```python
from build123d import *

# Parameters (mm, degrees)
SKETCH1_W           = 50
SKETCH1_H           = 50
BOSS_EXTRUDE1_DEPTH = 10
CUT_EXTRUDE3_DEPTH  = 6.3
SKETCH5_R           = 6.5
SKETCH5_R_2         = 3.1
BOSS_EXTRUDE2_DEPTH = 0.5
CUT_EXTRUDE4_DEPTH  = 57.789083458
FILLET2_R           = 5
CHAMFER2_SIZE       = 1
CHAMFER2_SIZE2      = 1.414213562
FILLET3_R           = 2
SKETCH9_R           = 3.1
CUT_EXTRUDE5_DEPTH  = 36.912254176
CHAMFER3_SIZE       = 1
SKETCH10_W          = 52
SKETCH10_H          = 19.709433282
CUT_EXTRUDE6_DEPTH  = 6.3
SKETCH14_R          = 3.25
CUT_EXTRUDE7_DEPTH  = 10
SKETCH15_W          = 4
SKETCH15_H          = 19.709433282
BOSS_EXTRUDE5_DEPTH = 6.3
SKETCH16_R          = 8
CUT_EXTRUDE8_DEPTH  = 10


with BuildPart() as part:
    # Sketch1 → Boss-Extrude1 (new body)
    with BuildSketch(Plane(origin=(0, 0, 0), x_dir=(1, 0, 0), z_dir=(0, 1, 0))):
        Rectangle(SKETCH1_W, SKETCH1_H)
    extrude(amount=BOSS_EXTRUDE1_DEPTH)

    # Sketch4 → Cut-Extrude3 (cut)
    with BuildSketch(Plane(origin=(0, 0, 0), x_dir=(-1, 0, 0), z_dir=(0, -1, 0))):
        with BuildLine():
            Line((21, -7.228416147), (21, -10.5))
            ThreePointArc((21, -10.5), (20.267766953, -12.267766953), (18.5, -13))
            Line((18.5, -13), (-18.5, -13))
            ThreePointArc((-18.5, -13), (-20.267766953, -12.267766953), (-21, -10.5))
            Line((-21, -10.5), (-21, -7.228416147))
            ThreePointArc((-21, -7.228416147), (-20.591644852, -6.017356006), (-19.533333333, -5.300838508))
            ThreePointArc((-19.533333333, -5.300838508), (-15.5, 0), (-19.533333333, 5.300838508))
            ThreePointArc((-19.533333333, 5.300838508), (-20.591644852, 6.017356006), (-21, 7.228416147))
            Line((-21, 7.228416147), (-21, 10.5))
            ThreePointArc((-21, 10.5), (-20.267766953, 12.267766953), (-18.5, 13))
            Line((-18.5, 13), (18.5, 13))
            ThreePointArc((18.5, 13), (20.267766953, 12.267766953), (21, 10.5))
            Line((21, 10.5), (21, 7.228416147))
            ThreePointArc((21, 7.228416147), (20.591644852, 6.017356006), (19.533333333, 5.300838508))
            ThreePointArc((19.533333333, 5.300838508), (15.5, 0), (19.533333333, -5.300838508))
            ThreePointArc((19.533333333, -5.300838508), (20.591644852, -6.017356006), (21, -7.228416147))
        make_face()
    extrude(amount=-CUT_EXTRUDE3_DEPTH, mode=Mode.SUBTRACT)

    # Sketch5 → Boss-Extrude2 (add)
    with BuildSketch(Plane(origin=(0, 6.3, 0), x_dir=(-1, 0, 0), z_dir=(0, -1, 0))):
        with Locations(Location((0, 0, 0), (0, 0, 90))):
            Circle(SKETCH5_R)
        with Locations(Location((0, 0, 0), (0, 0, 90))):
            Circle(SKETCH5_R_2, mode=Mode.SUBTRACT)
    extrude(amount=BOSS_EXTRUDE2_DEPTH)

    # Sketch8 → Cut-Extrude4 (cut, through all)
    with BuildSketch(Plane(origin=(25, 0, 0), x_dir=(0, 0, -1), z_dir=(1, 0, 0))):
        Polygon((-25, 0), (-25, 5), (-15.5, 5), (-20.5, 0), align=None)
        Polygon((25, 0), (25, 5), (15.5, 5), (20.5, 0), align=None)
    extrude(amount=-CUT_EXTRUDE4_DEPTH, mode=Mode.SUBTRACT)

    # Fillet2
    fillet2_edges = [part.edges().sort_by_distance(p)[0] for p in [
        (-25, 7.5, -25),
        (25, 7.5, -25),
        (25, 7.5, 25),
        (-25, 7.5, 25),
    ]]
    fillet(fillet2_edges, radius=FILLET2_R)

    # Chamfer2
    chamfer2_edges = [part.edges().sort_by_distance(p)[0] for p in [
        (0, 0, 20.5),
        (0, 0, -20.5),
    ]]
    chamfer2_side = [part.faces().sort_by_distance(p)[0] for p in [
        (24.353393474, 0, 0),
    ]]
    chamfer(chamfer2_edges, length=CHAMFER2_SIZE, length2=CHAMFER2_SIZE2, reference=chamfer2_side[0])

    # Fillet3
    fillet3_edges = [part.edges().sort_by_distance(p)[0] for p in [
        (25, 0.5, -19.5),
        (25, 0.5, 19.5),
        (-25, 0.5, -19.5),
        (-25, 0.5, 19.5),
    ]]
    fillet(fillet3_edges, radius=FILLET3_R)

    # Sketch9 → Cut-Extrude5 (cut, through all)
    with BuildSketch(Plane(origin=(0, 6.3, 0), x_dir=(-1, 0, 0), z_dir=(0, -1, 0))):
        with Locations(Location((0, 0, 0), (0, 0, 90))):
            Circle(SKETCH9_R)
    extrude(amount=-CUT_EXTRUDE5_DEPTH, mode=Mode.SUBTRACT)

    # Chamfer3
    chamfer3_edges = [part.edges().sort_by_distance(p)[0] for p in [
        (0, 10, 3.1),
    ]]
    chamfer(chamfer3_edges, length=CHAMFER3_SIZE)

    # Sketch10 → Cut-Extrude6 (cut)
    with BuildSketch(Plane.XZ):
        Rectangle(SKETCH10_W, SKETCH10_H)
    extrude(amount=-CUT_EXTRUDE6_DEPTH, mode=Mode.SUBTRACT)

    # Sketch14 → Cut-Extrude7 (cut)
    with BuildSketch(Plane.XZ.offset(-6.3)):
        with Locations(Location((15, 0, 0), (0, 0, 270))):
            Circle(SKETCH14_R)
        with Locations(Location((-15, 0, 0), (0, 0, 270))):
            Circle(SKETCH14_R)
    extrude(amount=-CUT_EXTRUDE7_DEPTH, mode=Mode.SUBTRACT)

    # Sketch15 → Boss-Extrude5 (add)
    with BuildSketch(Plane(origin=(0, 6.3, 0), x_dir=(-1, 0, 0), z_dir=(0, -1, 0))):
        with Locations((-23, 0)):
            Rectangle(SKETCH15_W, SKETCH15_H)
        with Locations((23, 0)):
            Rectangle(SKETCH15_W, SKETCH15_H)
    extrude(amount=BOSS_EXTRUDE5_DEPTH)

    # Sketch16 → Cut-Extrude8 (cut)
    with BuildSketch(Plane(origin=(0, 6.3, 0), x_dir=(-1, 0, 0), z_dir=(0, -1, 0))):
        with Locations((-15, 0)):
            Circle(SKETCH16_R)
        with Locations((15, 0)):
            Circle(SKETCH16_R)
    extrude(amount=CUT_EXTRUDE8_DEPTH, mode=Mode.SUBTRACT)


solid = part.part
```
Input: part model. Units: mm. Frame: model coordinates. A direction names the side the tool comes from. Round coordinates to 2 decimals unless told otherwise and drop trailing zeros. Order: outer loops, then holes, each group sorted by start corner. A loop starts at its lowest first (then second) coordinate and runs counter-clockwise, first axis right, second up. Notation, with made-up numbers: (3, 1) - (16, 1) arc R8 cw to (16, 6) - close; hole circle Ø10 at (16.5, 3). An arc over 180 degrees is marked (long way). Answer in a Markdown table with one row per item.
Item 1: Reachability of faces 4 (the flat face through (0, 5, 20)), 5 (the flat face through (0, 7, 25)), 6 (the cylindrical face through (-24.65, 0.85, 18.63)), 7 (the cylindrical face through (20.248, 3.106, 12.287)), 8 (the cylindrical face through (24.6, 0.9, -18.7)) from +Z, -Z, +X, -X, +Y, -Y: full face, straight path, thin tool, end or side. Return the list, or none.
Model answer:
| item | result |
|---|---|
| face 4 | +Z, +X, -X |
| face 5 | +Z, +X, -X, +Y, -Y |
| face 6 | +Z, -X, -Y |
| face 7 | -Y |
| face 8 | -Z, +X, -Y |
Item 2: Pin query (flat end, axial travel): pin 1 (5 mm diameter, centred on x = -15, z = 0, fed in from -Y); pin 2 (8 mm diameter, centred on x = 0, z = 0, fed in from +Y); pin 3 (1.9 mm diameter, centred on x = 7, y = 2, fed in from +Z); pin 4 (8 mm diameter, centred on x = -10, z = -2, fed in from -Y). Return the tip coordinate at first contact, or that it passes through.
Model answer:
| item | result |
|---|---|
| pin 1 | passes through |
| pin 2 | stops at y = 9.9 |
| pin 3 | stops at z = 19.45 |
| pin 4 | stops at y = 6.3 |
Item 3: Mould query, pull axis Z, two halves, no side actions, for faces 1 (the cylindrical face through (23, 8, 24)), 2 (the cylindrical face through (-23, 3, 0)), 3 (the flat face through (0.3, 3, -17.5)). Classes: released by +Z, released by -Z, zero draft, split by the parting line, or undercut.
Model answer:
| item | result |
|---|---|
| face 1 | released by +Z |
| face 2 | undercut |
| face 3 | released by -Z |
Item 4: Section query B-B (y = 8). Return the cut outline in (x, z).
Model answer:
| item | result |
|---|---|
| outline | (-25, -20) arc R5 ccw to (-20, -25) - (20, -25) arc R5 ccw to (25, -20) - (25, 20) arc R5 ccw to (20, 25) - (-20, 25) arc R5 ccw to (-25, 20) - close; hole circle Ø6.5 at (-15, 0); hole circle Ø6.2 at (0, 0); hole circle Ø6.5 at (15, 0) |
Item 5: Section query A-A (x = 0). Return the cut outline in (y, z).
Model answer:
| item | result |
|---|---|
| outline | (0, -19.5) - (1, -19.5) - (5, -15.5) - (5, -25) - (10, -25) - (10, -4.1) - (9, -3.1) - (6.3, -3.1) - (6.3, -13) - (0, -13) - close; (0, 13) - (6.3, 13) - (6.3, 3.1) - (9, 3.1) - (10, 4.1) - (10, 25) - (5, 25) - (5, 15.5) - (1, 19.5) - (0, 19.5) - close |
Item 6: Section query D-D (x = 11). Return the cut outline in (y, z).
Model answer:
| item | result |
|---|---|
| outline | (0, -19.5) - (1, -19.5) - (5, -15.5) - (5, -25) - (10, -25) - (10, 25) - (5, 25) - (5, 15.5) - (1, 19.5) - (0, 19.5) - (0, 13) - (6.3, 13) - (6.3, -13) - (0, -13) - close |
Item 7: Line query: line 1 (X direction, y = 8.45, z = 0); line 2 (Z direction, x = -18, y = 6); line 3 (X direction, y = 0.5, z = -9.5). Output: solid intervals per line, ascending.
Model answer:
| item | result |
|---|---|
| line 1 | x = -25 to -18.25, -11.75 to -3.1, 3.1 to 11.75, 18.25 to 25 |
| line 2 | z = -25 to -13, 13 to 25 |
| line 3 | x = -25 to -21, 21 to 25 |
Item 8: Section query C-C (z = 0). Return the cut outline in (x, y), then the cut area to 3 significant figures.
Model answer:
| item | result |
|---|---|
| outline | (-25, 0) - (-23, 0) - (-23, 6.3) - (-18.25, 6.3) - (-18.25, 10) - (-25, 10) - close; (-11.75, 6.3) - (-3.1, 6.3) - (-3.1, 9) - (-4.1, 10) - (-11.75, 10) - close; (3.1, 6.3) - (11.75, 6.3) - (11.75, 10) - (4.1, 10) - (3.1, 9) - close; (18.25, 6.3) - (23, 6.3) - (23, 0) - (25, 0) - (25, 10) - (18.25, 10) - close |
| area | 138 mm² |
